```python
from build123d import *

# Parameters (mm, degrees)
F1_DEPTH = 2
F0_R     = 3
F0_R_2   = 1.5
F2_DEPTH = 5
F4_DEPTH = 5
F5_DEPTH = 8
F6_DEPTH = 15
F7_DEPTH = 15
F3_W     = 1
F3_H     = 6
F8_DEPTH = 5


with BuildPart() as f1:
    # F0 (on Top) → F1 (new body)
    with BuildSketch(Plane.XY):
        with BuildLine():
            Line((-14, -20), (-2.7258296596, -20))
            ThreePointArc((-2.7258296596, -20), (0, -18.2529376149), (2.7258296596, -20))
            Line((2.7258296596, -20), (14, -20))
            ThreePointArc((14, -20), (14.7071067812, -19.7071067812), (15, -19))
            Line((15, -19), (15, -15.5))
            ThreePointArc((15, -15.5), (14.4142135624, -16.9142135624), (13, -17.5))
            Line((13, -17.5), (-13, -17.5))
            ThreePointArc((-13, -17.5), (-14.4142135624, -16.9142135624), (-15, -15.5))
            Line((-15, -15.5), (-15, -19))
            ThreePointArc((-15, -19), (-14.7071067812, -19.7071067812), (-14, -20))
        make_face()
    extrude(amount=F1_DEPTH)

    # F0 (on Top) → F2 (join)
    with BuildSketch(Plane.XY):
        with BuildLine():
            ThreePointArc((16.5, 20.5), (15.9142135624, 21.9142135624), (14.5, 22.5))
            Line((14.5, 22.5), (-16.5, 22.5))
            ThreePointArc((-16.5, 22.5), (-17.9142135624, 21.9142135624), (-18.5, 20.5))
            Line((-18.5, 20.5), (-18.5, 17.3358949354))
            Line((-18.5, 17.3358949354), (-18.5, -20.5))
            ThreePointArc((-18.5, -20.5), (-17.9142135624, -21.9142135624), (-16.5, -22.5))
            Line((-16.5, -22.5), (-2.7285225687, -22.5))
            ThreePointArc((-2.7285225687, -22.5), (-2.9999982596, -21.2497061259), (-2.7258296596, -20))
            Line((-2.7258296596, -20), (-14, -20))
            ThreePointArc((-14, -20), (-14.7071067812, -19.7071067812), (-15, -19))
            Line((-15, -19), (-15, -15.5))
            Line((-15, -15.5), (-15, 2.5))
            ThreePointArc((-15, 2.5), (-14.4142135624, 3.9142135624), (-13, 4.5))
            Line((-13, 4.5), (-12, 4.5))
            ThreePointArc((-12, 4.5), (-10.5857864376, 5.0857864376), (-10, 6.5))
            Line((-10, 6.5), (-10, 8.1054256072))
            ThreePointArc((-10, 8.1054256072), (-9.6405519552, 9.2493614806), (-8.6914107177, 9.9821118409))
            Line((-8.6914107177, 9.9821118409), (6.3085892823, 15.5084276303))
            ThreePointArc((6.3085892823, 15.5084276303), (8.1439358734, 15.2722933519), (9, 13.6317413967))
            Line((9, 13.6317413967), (9, 2.5))
            ThreePointArc((9, 2.5), (9.2928932188, 1.7928932188), (10, 1.5))
            Line((10, 1.5), (14, 1.5))
            ThreePointArc((14, 1.5), (14.7071067812, 1.2071067812), (15, 0.5))
            Line((15, 0.5), (15, -15.5))
            Line((15, -15.5), (15, -19))
            ThreePointArc((15, -19), (14.7071067812, -19.7071067812), (14, -20))
            Line((14, -20), (2.7258296596, -20))
            ThreePointArc((2.7258296596, -20), (2.9306559828, -20.6116455515), (3, -21.2529376149))
            ThreePointArc((3, -21.2529376149), (2.9313450587, -21.8910725121), (2.7285225687, -22.5))
            Line((2.7285225687, -22.5), (16.5, -22.5))
            ThreePointArc((16.5, -22.5), (17.9142135624, -21.9142135624), (18.5, -20.5))
            Line((18.5, -20.5), (18.5, 3.5))
            ThreePointArc((18.5, 3.5), (18.2071067812, 4.2071067812), (17.5, 4.5))
            ThreePointArc((17.5, 4.5), (16.7928932188, 4.7928932188), (16.5, 5.5))
            Line((16.5, 5.5), (16.5, 17.3358949354))
            Line((16.5, 17.3358949354), (16.5, 20.5))
        make_face()
        with BuildLine():
            ThreePointArc((-12.5, 17.3358949354), (-15.5, 14.3358949354), (-18.5, 17.3358949354))
            ThreePointArc((-18.5, 17.3358949354), (-15.5, 20.3358949354), (-12.5, 17.3358949354))
        make_face(mode=Mode.SUBTRACT)
        with Locations((13.5, 17.3358949354)):
            Circle(F0_R, mode=Mode.SUBTRACT)
        with BuildLine():
            ThreePointArc((-2.7258296596, -20), (-2.9999982596, -21.2497061259), (-2.7285225687, -22.5))
            Line((-2.7285225687, -22.5), (-0.8335678783, -22.5))
            ThreePointArc((-0.8335678783, -22.5), (-1.4999905856, -21.2476231938), (-0.8247104541, -20))
            Line((-0.8247104541, -20), (-2.7258296596, -20))
        make_face()
        with BuildLine():
            Line((-0.8335678783, -22.5), (-2.7285225687, -22.5))
            ThreePointArc((-2.7285225687, -22.5), (0, -24.2529376149), (2.7285225687, -22.5))
            Line((2.7285225687, -22.5), (0.8335678783, -22.5))
            ThreePointArc((0.8335678783, -22.5), (0, -22.7529376149), (-0.8335678783, -22.5))
        make_face()
        with BuildLine():
            Line((0.8335678783, -22.5), (2.7285225687, -22.5))
            ThreePointArc((2.7285225687, -22.5), (2.9313450587, -21.8910725121), (3, -21.2529376149))
            ThreePointArc((3, -21.2529376149), (2.9306559828, -20.6116455515), (2.7258296596, -20))
            Line((2.7258296596, -20), (0.8247104541, -20))
            ThreePointArc((0.8247104541, -20), (1.3204290366, -20.5412725537), (1.5, -21.2529376149))
            ThreePointArc((1.5, -21.2529376149), (1.3229421411, -21.9599199989), (0.8335678783, -22.5))
        make_face()
        with BuildLine():
            ThreePointArc((2.7258296596, -20), (0, -18.2529376149), (-2.7258296596, -20))
            Line((-2.7258296596, -20), (-0.8247104541, -20))
            ThreePointArc((-0.8247104541, -20), (0, -19.7529376149), (0.8247104541, -20))
            Line((0.8247104541, -20), (2.7258296596, -20))
        make_face()
        with BuildLine():
            ThreePointArc((-12.5, 17.3358949354), (-15.5, 20.3358949354), (-18.5, 17.3358949354))
            ThreePointArc((-18.5, 17.3358949354), (-15.5, 14.3358949354), (-12.5, 17.3358949354))
        make_face()
        with Locations((-15.5, 17.3358949354)):
            Circle(F0_R_2, mode=Mode.SUBTRACT)
        with Locations((13.5, 17.3358949354)):
            Circle(F0_R)
        with Locations((13.5, 17.3358949354)):
            Circle(F0_R_2, mode=Mode.SUBTRACT)
    extrude(amount=F2_DEPTH)

    # F3 (on face) → F4 (join)
    with BuildSketch(Plane.XY.offset(5)):
        with BuildLine():
            ThreePointArc((-18.5, -14.5), (-18.2071067812, -15.2071067812), (-17.5, -15.5))
            Line((-17.5, -15.5), (-16, -15.5))
            ThreePointArc((-16, -15.5), (-15.2928932188, -15.2071067812), (-15, -14.5))
            Line((-15, -14.5), (-15, 2.5))
            ThreePointArc((-15, 2.5), (-14.4142135624, 3.9142135624), (-13, 4.5))
            Line((-13, 4.5), (-12, 4.5))
            ThreePointArc((-12, 4.5), (-10.5857864376, 5.0857864376), (-10, 6.5))
            Line((-10, 6.5), (-10, 8.1054256072))
            ThreePointArc((-10, 8.1054256072), (-9.6405519552, 9.2493614806), (-8.6914107177, 9.9821118409))
            Line((-8.6914107177, 9.9821118409), (-11.5, 8.9473684211))
            Line((-11.5, 8.9473684211), (-11.5, 8.5))
            ThreePointArc((-11.5, 8.5), (-11.7928932188, 7.7928932188), (-12.5, 7.5))
            Line((-12.5, 7.5), (-16.5, 7.5))
            ThreePointArc((-16.5, 7.5), (-17.9142135624, 6.9142135624), (-18.5, 5.5))
            Line((-18.5, 5.5), (-18.5, -14.5))
        make_face()
    extrude(amount=F4_DEPTH)

    # F3 (on face) → F5 (join)
    with BuildSketch(Plane.XY.offset(5)):
        with BuildLine():
            Line((4.5, 22.5), (-9.5, 22.5))
            ThreePointArc((-9.5, 22.5), (-10.9142135624, 21.9142135624), (-11.5, 20.5))
            Line((-11.5, 20.5), (-11.5, 8.9473684211))
            Line((-11.5, 8.9473684211), (-8.6914107177, 9.9821118409))
            Line((-8.6914107177, 9.9821118409), (6.3085892823, 15.5084276303))
            Line((6.3085892823, 15.5084276303), (6.5, 15.5789473684))
            Line((6.5, 15.5789473684), (6.5, 20.5))
            ThreePointArc((6.5, 20.5), (5.9142135624, 21.9142135624), (4.5, 22.5))
        make_face()
    extrude(amount=F5_DEPTH)

    # F3 (on face) → F6 (join)
    with BuildSketch(Plane.XY.offset(5)):
        with BuildLine():
            ThreePointArc((9, -21.5), (9.2928932188, -22.2071067812), (10, -22.5))
            Line((10, -22.5), (16.5, -22.5))
            ThreePointArc((16.5, -22.5), (17.9142135624, -21.9142135624), (18.5, -20.5))
            ThreePointArc((18.5, -20.5), (18.2071067812, -19.7928932188), (17.5, -19.5))
            Line((17.5, -19.5), (14.8660254038, -19.5))
            ThreePointArc((14.8660254038, -19.5), (14.5, -19.8660254038), (14, -20))
            Line((14, -20), (9.1339745962, -20))
            ThreePointArc((9.1339745962, -20), (9.0340741737, -20.2411809549), (9, -20.5))
            Line((9, -20.5), (9, -21.5))
        make_face()
        with BuildLine():
            ThreePointArc((10, -19.5), (9.5, -19.6339745962), (9.1339745962, -20))
            Line((9.1339745962, -20), (14, -20))
            ThreePointArc((14, -20), (14.5, -19.8660254038), (14.8660254038, -19.5))
            Line((14.8660254038, -19.5), (10, -19.5))
        make_face()
    extrude(amount=F6_DEPTH)

    # F3 (on face) → F7 (join)
    with BuildSketch(Plane.XY.offset(5)):
        with BuildLine():
            ThreePointArc((15.5, 10.5), (16.2071067812, 10.7928932188), (16.5, 11.5))
            ThreePointArc((16.5, 11.5), (16.2071067812, 12.2071067812), (15.5, 12.5))
            Line((15.5, 12.5), (10, 12.5))
            ThreePointArc((10, 12.5), (9.2928932188, 12.2071067812), (9, 11.5))
            ThreePointArc((9, 11.5), (9.2928932188, 10.7928932188), (10, 10.5))
            Line((10, 10.5), (12.25, 10.5))
            Line((12.25, 10.5), (13.25, 10.5))
            Line((13.25, 10.5), (15.5, 10.5))
        make_face()
        with BuildLine():
            ThreePointArc((17.5, 1.5), (18.2071067812, 1.7928932188), (18.5, 2.5))
            Line((18.5, 2.5), (18.5, 3.5))
            ThreePointArc((18.5, 3.5), (18.2071067812, 4.2071067812), (17.5, 4.5))
            Line((17.5, 4.5), (13.25, 4.5))
            Line((13.25, 4.5), (12.25, 4.5))
            Line((12.25, 4.5), (10, 4.5))
            ThreePointArc((10, 4.5), (9.2928932188, 4.2071067812), (9, 3.5))
            Line((9, 3.5), (9, 2.5))
            ThreePointArc((9, 2.5), (9.2928932188, 1.7928932188), (10, 1.5))
            Line((10, 1.5), (14, 1.5))
            Line((14, 1.5), (17.5, 1.5))
        make_face()
    extrude(amount=F7_DEPTH)

    # F3 (on face) → F8 (join)
    with BuildSketch(Plane.XY.offset(5)):
        with Locations((12.75, 7.5)):
            Rectangle(F3_W, F3_H)
        with BuildLine():
            ThreePointArc((17.5, -19.5), (18.2071067812, -19.7928932188), (18.5, -20.5))
            Line((18.5, -20.5), (18.5, 2.5))
            ThreePointArc((18.5, 2.5), (18.2071067812, 1.7928932188), (17.5, 1.5))
            Line((17.5, 1.5), (14, 1.5))
            ThreePointArc((14, 1.5), (14.7071067812, 1.2071067812), (15, 0.5))
            Line((15, 0.5), (15, -19))
            ThreePointArc((15, -19), (14.9659258263, -19.2588190451), (14.8660254038, -19.5))
            Line((14.8660254038, -19.5), (17.5, -19.5))
        make_face()
    extrude(amount=F8_DEPTH)


solid = f1.part
```
Here's how the part is built. I have some questions about the finished solid (model axes, mm). A direction names the side the tool comes from. Coordinates: 2 decimals unless noted, no trailing zeros. Write each loop counter-clockwise with the first axis right and the second up, starting at its lowest first coordinate (ties: lowest second). Pieces come first, ordered by that corner, then holes. Notation, with made-up numbers: (-32, -18) -> (-24, -18) arc R12 cw to (-24, 3) -> close; hole circle Ø6 at (16, 20). An arc over 180 degrees is marked (long way). Use a Markdown table: item, result. Add a question column.
(1) If we section it at A-A, the plane y = -7.5: Write out the boundary of the cut face in (x, z).
(2) If we section it at D-D, the plane y = 15: Write out the boundary of the cut face in (x, z).
(3) We'd pull the mould along Y, two halves only. Please class faces 4 (the flat face through (-17, -15.5, 7)), 5 (the cylindrical face through (-14.699, -19.715, 3.479)), 6 (the cylindrical face through (-17.9, 21.93, 2.46)), 7 (the flat face through (12.25, 7, 7)): +Y half, -Y half, draft (parallel to the pull), parting line (faces both ways), or undercut.
(4) If we section it at C-C, the plane z = 15: Write out the boundary of the cut face in (x, y).
(5) I'm going to push flat-ended pins straight in: P1, Ø12, axis at x = 7, z = 8.5, coming from the +Y side; P2, Ø8, axis at x = -3, y = -21, coming from the +Z side; P3, Ø2, axis at x = 2.5, y = -18, coming from the +Z side; P4, Ø1.5, axis at y = 15, z = 5.5, coming from the +X side. Where does each tip first touch, or does it pass through?
(6) Please list where these lines run through material, in increasing order: line 1 (Y direction, x = 14, z = 8.75); line 2 (Y direction, x = 13.5, z = 2.1); line 3 (Y direction, x = 7, z = 4).
(7) If we section it at B-B, the plane x = 11: Write out the boundary of the cut face in (y, z), and give its area (4 significant figures).
(8) For faces 1 (the cylindrical face through (9.285, -22.199, 12.395)), 2 (the cylindrical face through (0.048, -18.253, 3.479)), 3 (the cylindrical face through (-9.65, 9.235, 4.93)), which set-ups out of +Z, -Z, +X, -X, +Y, -Y let a thin tool reach every point of the face, with its end or its side?
Outcome:
| question | item | result |
|---|---|---|
| 1 | outline | (-18.5, 0) -> (-15, 0) -> (-15, 10) -> (-18.5, 10) -> close; (15, 0) -> (18.5, 0) -> (18.5, 10) -> (15, 10) -> close |
| 2 | outline | (-18.5, 0) -> (4.93, 0) -> (4.93, 13) -> (-11.5, 13) -> (-11.5, 5) -> (-18.5, 5) -> close; (8.46, 0) -> (16.5, 0) -> (16.5, 5) -> (8.46, 5) -> close |
| 3 | face 4 | -Y half |
| 3 | face 5 | undercut |
| 3 | face 6 | +Y half |
| 3 | face 7 | undercut |
| 4 | outline | (9, -21.5) arc R1 ccw to (10, -22.5) -> (16.5, -22.5) arc R2 ccw to (18.5, -20.5) arc R1 ccw to (17.5, -19.5) -> (10, -19.5) arc R1 ccw to (9, -20.5) -> close; (9, 2.5) arc R1 ccw to (10, 1.5) -> (17.5, 1.5) arc R1 ccw to (18.5, 2.5) -> (18.5, 3.5) arc R1 ccw to (17.5, 4.5) -> (10, 4.5) arc R1 ccw to (9, 3.5) -> close; (10, 10.5) -> (15.5, 10.5) arc R1 ccw to (15.5, 12.5) -> (10, 12.5) arc R1 ccw to start |
| 5 | P1 | stops at y = 22.5 |
| 5 | P2 | stops at z = 5 |
| 5 | P3 | stops at z = 2 |
| 5 | P4 | stops at x = 16.5 |
| 6 | line 1 | y = -22.5 to -19.5, 1.5 to 4.5, 10.5 to 12.5 |
| 6 | line 2 | y = -22.5 to -20, 1.5 to 15.84, 18.84 to 22.5 |
| 6 | line 3 | y = -22.5 to -20, 15.63 to 22.5 |
| 7 | outline | (-22.5, 0) -> (-17.5, 0) -> (-17.5, 2) -> (-20, 2) -> (-20, 5) -> (-19.5, 5) -> (-19.5, 20) -> (-22.5, 20) -> close; (1.5, 0) -> (22.5, 0) -> (22.5, 5) -> (12.5, 5) -> (12.5, 20) -> (10.5, 20) -> (10.5, 5) -> (4.5, 5) -> (4.5, 20) -> (1.5, 20) -> close |
| 7 | area | 242.5 mm^2 |
| 8 | face 1 | +Z, -X, -Y |
| 8 | face 2 | +Z |
| 8 | face 3 | +Z, -Z |
